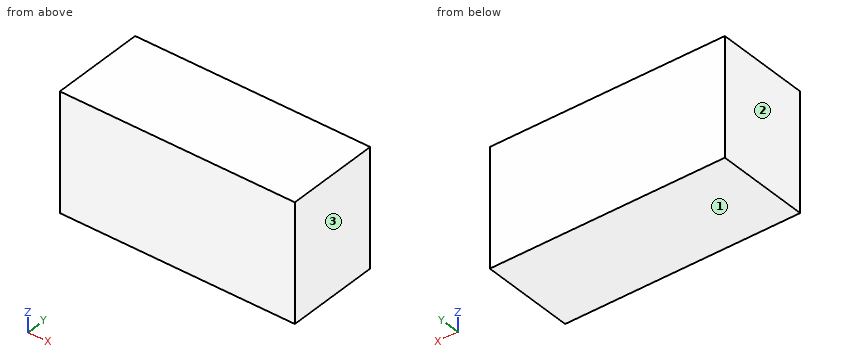
from build123d import *

# Parameters (mm, degrees)
F0_W     = 254
F0_H     = 127
F1_DEPTH = 101.6
F2_T     = -2.54
F3_W     = 248.92
F3_H     = 121.92
F4_DEPTH = 2.54


with BuildPart() as f1:
    # F0 (on Front) → F1 (new body)
    with BuildSketch(Plane.XZ):
        Rectangle(F0_W, F0_H)
    extrude(amount=-F1_DEPTH)

    # F2
    f2_openings = [f1.faces().sort_by_distance(p)[0] for p in [
        (0, 0, 0),
    ]]
    offset(amount=F2_T, openings=f2_openings)

    # F3 (on face) → F4 (join)
    with BuildSketch(Plane.XZ):
        Rectangle(F3_W, F3_H)
    extrude(amount=-F4_DEPTH)


solid = f1.part
Here's how the part is built. I have some questions about the finished solid (model axes, mm). Face numbers are marked on the shaded views. Coordinates: 2 decimals unless noted, no trailing zeros. Loops run counter-clockwise (first coordinate to the right, second up) from the corner with the lowest first, then second, coordinate; pieces in that order, holes last.
1. If we mould it in two halves opening along X, with no side actions, what happens to the marked faces 1, 2 and 3? For each: pulls with the +X half, pulls with the -X half, needs draft (parallel to the pull), parting line crosses it, or undercut.
2. I need wall thicknesses on L1, parallel to X at y = 49, z = -5; L2, parallel to Z at x = 71, y = 47; L3, parallel to Y at x = 70, z = 7.5. Which ranges of each line are inside material? Lowest first, please.
3. Imagine slicing it at B-B, the plane x = -50. Please give me the cut outline in (y, z), and give its area (3 significant figures).
4. Imagine slicing it at A-A, the plane y = 55. Please give me the cut outline in (x, z).
Taken from the geometry:
1. face 1: needs draft
1. face 2: pulls with the -X half
1. face 3: pulls with the +X half
2. L1: x = -127 to -124.46, 124.46 to 127
2. L2: z = -63.5 to -60.96, 60.96 to 63.5
2. L3: y = 0 to 2.54, 99.06 to 101.6
3. outline: (0, -63.5) - (101.6, -63.5) - (101.6, 63.5) - (0, 63.5) - close; hole (2.54, -60.96) - (99.06, -60.96) - (99.06, 60.96) - (2.54, 60.96) - close
3. area: 1,140 mm2
4. outline: (-127, -63.5) - (127, -63.5) - (127, 63.5) - (-127, 63.5) - close; hole (-124.46, -60.96) - (124.46, -60.96) - (124.46, 60.96) - (-124.46, 60.96) - close
